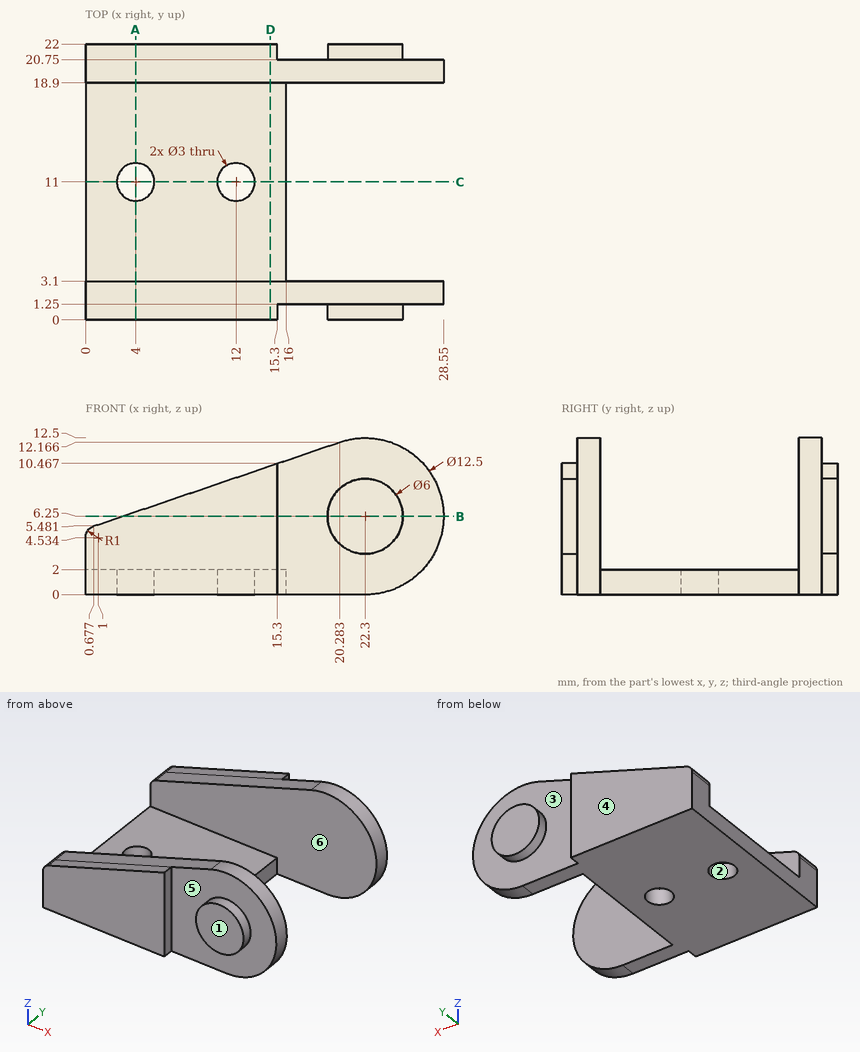
Source: three-view drawing plus pictorial views. Frame: mm from the lowest corner of the part. A direction names the side the tool comes from. Coordinates: 2 decimals unless noted, no trailing zeros. Loops run counter-clockwise (first coordinate to the right, second up) from the corner with the lowest first, then second, coordinate; pieces in that order, holes last. Notation, with made-up numbers: (7, 49.25) -> (49, 49.25) arc R19 cw to (49, 55.25) -> close; hole circle Ø7 at (54, 56.5). An arc over 180 degrees is marked (long way). One line per item, written item: value.
(1) Cut plane B-B (z = 6.25). Output: boundary loops of the cut face in (x, y), then the cut area to 3 significant figures.
Answer below:
outline: (2.93, 0) -> (15.3, 0) -> (15.3, 1.25) -> (19.3, 1.25) -> (19.3, 0) -> (25.3, 0) -> (25.3, 1.25) -> (28.55, 1.25) -> (28.55, 3.1) -> (2.93, 3.1) -> close; (2.93, 18.9) -> (28.55, 18.9) -> (28.55, 20.75) -> (25.3, 20.75) -> (25.3, 22) -> (19.3, 22) -> (19.3, 20.75) -> (15.3, 20.75) -> (15.3, 22) -> (2.93, 22) -> close
area: 141 mm2
(2) Cut plane C-C (y = 11). Output: boundary loops of the cut face in (x, z), then the cut area to 3 significant figures.
Answer below:
outline: (0, 0) -> (2.5, 0) -> (2.5, 2) -> (0, 2) -> close; (5.5, 0) -> (10.5, 0) -> (10.5, 2) -> (5.5, 2) -> close; (13.5, 0) -> (16, 0) -> (16, 2) -> (13.5, 2) -> close
area: 20.0 mm2
(3) Pin query (flat end, axial travel): pin 1 Ø1.6 at (y, z) = (11.5, 1) entering from +X; pin 2 Ø1 at (y, z) = (0.5, 6.5) entering from +X; pin 3 Ø12.5 at (x, y) = (6, 11) entering from +Z; pin 4 Ø0.6 at (y, z) = (21, 6) entering from +X. Return the tip coordinate at first contact, or that it passes through.
Answer below:
pin 1: stops at x = 16
pin 2: stops at x = 25.3
pin 3: stops at z = 2
pin 4: stops at x = 28.55
(4) Cut plane A-A (x = 4). Output: boundary loops of the cut face in (y, z).
Answer below:
outline: (0, 0) -> (9.5, 0) -> (9.5, 2) -> (3.1, 2) -> (3.1, 6.61) -> (0, 6.61) -> close; (12.5, 0) -> (22, 0) -> (22, 6.61) -> (18.9, 6.61) -> (18.9, 2) -> (12.5, 2) -> close
(5) Ray query, line 1 along Y through (x, z) = (17, 7.25); line 2 along Y through (x, z) = (4, 0.95); line 3 along X through (y, z) = (3.75, 1). Return the intervals inside material, ascending.
Answer below:
line 1: y = 1.25 to 3.1, 18.9 to 20.75
line 2: y = 0 to 9.5, 12.5 to 22
line 3: x = 0 to 16
(6) Set-up query: the marked faces 4, 5 and 6. Return all of +Z, -Z, +X, -X, +Y, -Y with unobstructed straight access to the full face (end or side cutting, diameter ignored); none if empty.
Answer below:
face 4: +Z, -Z, +X, -X, +Y
face 5: -Y
face 6: +Z, +X
(7) Cut plane D-D (x = 14.75). Output: boundary loops of the cut face in (y, z).
Answer below:
outline: (0, 0) -> (22, 0) -> (22, 10.28) -> (18.9, 10.28) -> (18.9, 2) -> (3.1, 2) -> (3.1, 10.28) -> (0, 10.28) -> close
(8) Draft query along Y for the marked faces 1, 2 and 3. Return one class per face: pulls with the +Y half, pulls with the -Y half, needs draft (parallel to the pull), parting line crosses it, or undercut.
Answer below:
face 1: pulls with the -Y half
face 2: undercut
face 3: pulls with the +Y half
